```python
from build123d import *

# Parameters (mm, degrees)
F0_R     = 5.2
F1_DEPTH = 4
F2_DEPTH = 4


with BuildPart() as f1:
    # F0 (on Top) → F1 (new body)
    with BuildSketch(Plane.XY):
        Polygon((40.4145188433, 70), (-40.4145188433, 70), (-80.8290376865, 0), (-40.4145188433, -70), (40.4145188433, -70), (80.8290376865, 0), align=None)
        with Locations((-35, -60.6217782649)):
            Circle(F0_R, mode=Mode.SUBTRACT)
        with Locations((35, -60.6217782649)):
            Circle(F0_R, mode=Mode.SUBTRACT)
        with Locations((-70, 0)):
            Circle(F0_R, mode=Mode.SUBTRACT)
        with Locations((-35, 60.6217782649)):
            Circle(F0_R, mode=Mode.SUBTRACT)
        with Locations((70, 0)):
            Circle(F0_R, mode=Mode.SUBTRACT)
        with Locations((35, 60.6217782649)):
            Circle(F0_R, mode=Mode.SUBTRACT)
        with Locations((-70, 0)):
            Circle(F0_R)
        with Locations((-35, 60.6217782649)):
            Circle(F0_R)
        with Locations((35, 60.6217782649)):
            Circle(F0_R)
        with Locations((70, 0)):
            Circle(F0_R)
        with Locations((35, -60.6217782649)):
            Circle(F0_R)
        with Locations((-35, -60.6217782649)):
            Circle(F0_R)
    extrude(amount=-F1_DEPTH)

    # F0 (on Top) → F2 (join)
    with BuildSketch(Plane.XY):
        Polygon((40.4145188433, 70), (-40.4145188433, 70), (-80.8290376865, 0), (-40.4145188433, -70), (40.4145188433, -70), (80.8290376865, 0), align=None)
        with Locations((-35, -60.6217782649)):
            Circle(F0_R, mode=Mode.SUBTRACT)
        with Locations((35, -60.6217782649)):
            Circle(F0_R, mode=Mode.SUBTRACT)
        with Locations((-70, 0)):
            Circle(F0_R, mode=Mode.SUBTRACT)
        with Locations((-35, 60.6217782649)):
            Circle(F0_R, mode=Mode.SUBTRACT)
        with Locations((70, 0)):
            Circle(F0_R, mode=Mode.SUBTRACT)
        with Locations((35, 60.6217782649)):
            Circle(F0_R, mode=Mode.SUBTRACT)
    extrude(amount=F2_DEPTH)


solid = f1.part
```
CAD build for the part. Positions are in the model's coordinates, mm. A direction names the side the tool comes from. Coordinates: 2 decimals unless noted, no trailing zeros. Write each loop counter-clockwise with the first axis right and the second up, starting at its lowest first coordinate (ties: lowest second). Pieces come first, ordered by that corner, then holes. Notation, with made-up numbers: (9, -15) -> (37, -15) arc R5 cw to (37, -10) -> close; hole circle Ø2 at (5.5, 16.25). An arc over 180 degrees is marked (long way). Use CSV: the item, a comma, the result in double quotes. Start each with the question number.
Item 1: Two-plate mould, pull along X, no slides. Class faces 3 (the flat face through (35, 61, 0)), 4 (the flat face through (60.34, -35.49, -0.06)), 5 (the flat face through (1, 70, 0)): +X half, -X half, draft (parallel to the pull), parting line (faces both ways), or undercut.
Item 2: Band-saw the part on B-B, the plane z = 2.25. Write the cut outline in (x, y).
Item 3: Band-saw the part on C-C, the plane y = 25. Write the cut outline in (x, z), plus the area to 3 significant figures.
Item 4: Band-saw the part on D-D, the plane x = -70. Write the cut outline in (y, z), plus the area to 3 significant figures.
Item 5: Tool access for faces 1 (the flat face through (60.905, 34.51, -0.056)), 2 (the flat face through (35, -61, 0)): list every direction of +Z, -Z, +X, -X, +Y, -Y with a clear straight run to the whole face (end or side of a thin tool).
Item 6: Band-saw the part on A-A, the plane x = -35. Write the cut outline in (y, z), plus the area to 3 significant figures.
Item 7: Drop flat-ended pins along their axis: P1, Ø11.5, axis at x = 68, y = -1.5, coming from the +Z side; P2, Ø5, axis at x = 34, y = 62.5, coming from the +Z side; P3, Ø3, axis at x = -57.5, z = -3, coming from the -Y side; P4, Ø1, axis at y = 48, z = 1.5, coming from the +X side. Give the stop position or say it passes through.
Item 8: Wall check: probe 1 along Y at (x, z) = (35, 2.7); probe 2 along X at (y, z) = (-1, 2.5); probe 3 along X at (y, z) = (-57.5, 2). Give the ranges that are in metal, low to high.
Response values:
1,face 3,"undercut"
1,face 4,"+X half"
1,face 5,"draft"
2,outline,"(-80.83, 0) -> (-40.41, -70) -> (40.41, -70) -> (80.83, 0) -> (40.41, 70) -> (-40.41, 70) -> close; hole circle Ø10.4 at (-70, 0); hole circle Ø10.4 at (-35, -60.62); hole circle Ø10.4 at (-35, 60.62); hole circle Ø10.4 at (35, -60.62); hole circle Ø10.4 at (35, 60.62); hole circle Ø10.4 at (70, 0)"
3,outline,"(-66.4, -4) -> (66.4, -4) -> (66.4, 4) -> (-66.4, 4) -> close"
3,area,"1,060 mm2"
4,outline,"(-18.76, -4) -> (18.76, -4) -> (18.76, 4) -> (5.2, 4) -> (5.2, 0) -> (-5.2, 0) -> (-5.2, 4) -> (-18.76, 4) -> close"
4,area,"259 mm2"
5,face 1,"+Z, -Z, +X, +Y"
5,face 2,"+Z"
6,outline,"(-70, -4) -> (70, -4) -> (70, 4) -> (65.82, 4) -> (65.82, 0) -> (55.42, 0) -> (55.42, 4) -> (-55.42, 4) -> (-55.42, 0) -> (-65.82, 0) -> (-65.82, 4) -> (-70, 4) -> close"
6,area,"1,040 mm2"
7,P1,"stops at z = 4"
7,P2,"stops at z = 0"
7,P3,"stops at y = -43.01"
7,P4,"stops at x = 53.4"
8,probe 1,"y = -70 to -65.82, -55.42 to 55.42, 65.82 to 70"
8,probe 2,"x = -80.25 to -75.1, -64.9 to 64.9, 75.1 to 80.25"
8,probe 3,"x = -47.63 to -39.16, -30.84 to 30.84, 39.16 to 47.63"
